Design review of the part shown in the three views and the two pictorial views. Dimensions are in mm from the part's minimum x, y and z. Round coordinates to 2 decimals unless told otherwise and drop trailing zeros. Order: outer loops, then holes, each group sorted by start corner. A loop starts at its lowest first (then second) coordinate and runs counter-clockwise, first axis right, second up.
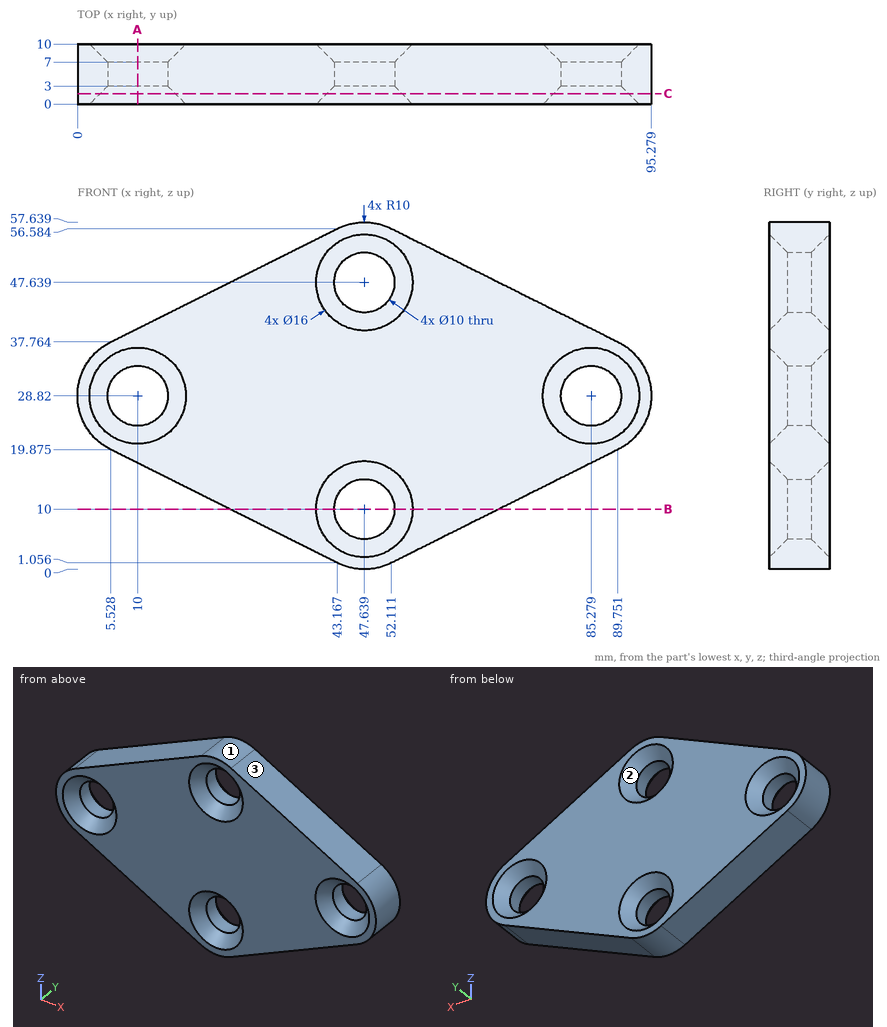
1) To check wall thickness, follow line 1 along X through (y, z) = (8.25, 33.5) (1 decimal); line 2 along X through (y, z) = (3.5, 30); line 3 along Z through (x, y) = (44, 8.5) (1 decimal). State the ranges of each line that lie inside material, in increasing order.
Results:
line 1: x = 1.2 to 5.9, 14.1 to 81.1, 89.4 to 94.1
line 2: x = 0.07 to 5.14, 14.86 to 80.42, 90.14 to 95.21
line 3: z = 0.7 to 4.6, 15.4 to 42.3, 53 to 57
2) Take a section at C-C on y = 1.75. State how many separate pieces and enclosed holes the cut face has, plus the area to 3 significant figures.
Results:
separate pieces: 1
enclosed holes: 4
area: 2,920 mm2
3) Take a section at A-A on x = 10. Give the boundary of the cut face in (y, z).
Results:
outline: (0, 17.64) - (10, 17.64) - (10, 20.82) - (7, 23.82) - (3, 23.82) - (0, 20.82) - close; (0, 36.82) - (3, 33.82) - (7, 33.82) - (10, 36.82) - (10, 40) - (0, 40) - close
4) The part is to be moulded in two halves that separate along X. For the marked faces 1, 2 and 3, say which applies: released by +X, released by -X, zero draft, split by the parting line, or undercut.
Results:
face 1: split by the parting line
face 2: undercut
face 3: released by +X
5) Take a section at B-B on z = 10. Give the boundary of the cut face in (x, y).
Results:
outline: (25.28, 0) - (39.64, 0) - (42.64, 3) - (42.64, 7) - (39.64, 10) - (25.28, 10) - close; (52.64, 3) - (55.64, 0) - (70, 0) - (70, 10) - (55.64, 10) - (52.64, 7) - close
6) Clearance check with flat-ended pins moving along their axes: P1, Ø11.5, axis at x = 47.64, z = 47.64, coming from the +Y side; P2, Ø6, axis at x = 85.28, z = 28.82, coming from the +Y side; P3, Ø2, axis at x = 42.5, y = 5.5, coming from the +Z side; P4, Ø1, axis at y = 2, z = 48.5, coming from the +X side. State where each tip first meets the part, or that it passes through.
Results:
P1: stops at y = 7.75
P2: passes through
P3: stops at z = 56.74
P4: stops at x = 69.28
